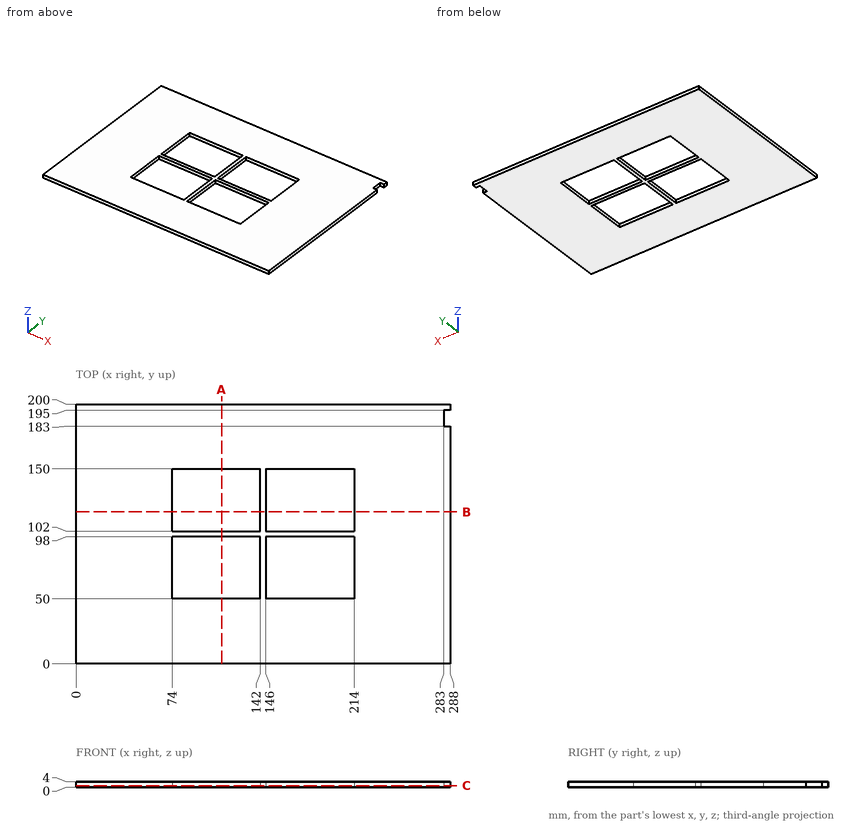
Drawing for the job (mm, zero at the part's lowest x, y, z). Give positions to 0.01 mm unless a question says otherwise; leave off trailing zeros. Write each loop counter-clockwise with the first axis right and the second up, starting at its lowest first coordinate (ties: lowest second). Pieces come first, ordered by that corner, then holes. Notation, with made-up numbers: (9, 6) -> (32, 6) arc R13 ccw to (32, 21) -> close; hole circle Ø5 at (65.25, 28). An arc over 180 degrees is marked (long way). Put each result on its own line as item: value. Start each with the question number.
Item 1: Cut at A-A (x = 112). List the corners of the cut face in (y, z), then the cut area to 3 significant figures.
Item 2: Cut at C-C (z = 1). List the corners of the cut face in (x, y), then the cut area to 3 significant figures.
Item 3: Cut at B-B (y = 117). List the corners of the cut face in (x, z), then the cut area to 3 significant figures.
Item 4: Wall check: L1, parallel to Y at x = 152.5, z = 1.7; L2, parallel to X at y = 111.5, z = 3.8; L3, parallel to X at y = 190, z = 2.85. Give the ranges that are in metal, low to high. Write a range as [from, to].
Answer list:
1. outline: (0, 0) -> (50, 0) -> (50, 4) -> (0, 4) -> close; (98, 0) -> (102, 0) -> (102, 4) -> (98, 4) -> close; (150, 0) -> (200, 0) -> (200, 4) -> (150, 4) -> close
1. area: 416 mm2
2. outline: (0, 0) -> (288, 0) -> (288, 183) -> (283, 183) -> (283, 195) -> (288, 195) -> (288, 200) -> (0, 200) -> close; hole (74, 50) -> (142, 50) -> (142, 98) -> (74, 98) -> close; hole (74, 102) -> (142, 102) -> (142, 150) -> (74, 150) -> close; hole (146, 50) -> (214, 50) -> (214, 98) -> (146, 98) -> close; hole (146, 102) -> (214, 102) -> (214, 150) -> (146, 150) -> close
2. area: 44,500 mm2
3. outline: (0, 0) -> (74, 0) -> (74, 4) -> (0, 4) -> close; (142, 0) -> (146, 0) -> (146, 4) -> (142, 4) -> close; (214, 0) -> (288, 0) -> (288, 4) -> (214, 4) -> close
3. area: 608 mm2
4. L1: y = [0, 50], [98, 102], [150, 200]
4. L2: x = [0, 74], [142, 146], [214, 288]
4. L3: x = [0, 283]
